Can you work these out from the model? Positions are in its coordinate system, mm. Face numbers are marked on the shaded views. A direction names the side the tool comes from. Round coordinates to 2 decimals unless told otherwise and drop trailing zeros. Loops run counter-clockwise (first coordinate to the right, second up) from the corner with the lowest first, then second, coordinate; pieces in that order, holes last. Notation, with made-up numbers: (33.25, 64) -> (53.25, 64) arc R24 cw to (53.25, 85) -> close; hole circle Ø4 at (-3.5, 52). An arc over 180 degrees is marked (long way). Answer as a JSON object with one key per item and string values.
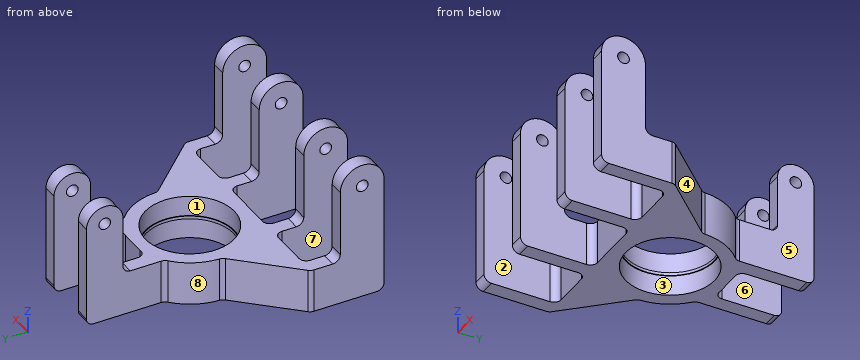
```python
from build123d import *

# Parameters (mm, degrees)
BOSS_EXTRUDE2_DEPTH     = 30
SKETCH2_R               = 4
BOSS_EXTRUDE3_DEPTH     = 10
CUT_EXTRUDE3_DEPTH      = 162
SKETCH4_R               = 4
BOSS_EXTRUDE4_DEPTH     = 10
SKETCH5_R               = 4
BOSS_EXTRUDE5_DEPTH     = 10
SKETCH6_R               = 4
BOSS_EXTRUDE6_DEPTH     = 10
SKETCH7_R               = 4
BOSS_EXTRUDE7_DEPTH     = 10
CUT_EXTRUDE4_DEPTH      = 167.226502099
CUT_EXTRUDE4_DEPTH_BACK = 57
SKETCH13_R              = 4
BOSS_EXTRUDE8_DEPTH     = 10
SKETCH14_R              = 30
CUT_EXTRUDE5_DEPTH      = 136.392946641
SKETCH15_R              = 30.5
CUT_EXTRUDE6_DEPTH      = 14
CUT_EXTRUDE7_START      = -14
SKETCH16_R              = 30.5
CUT_EXTRUDE7_DEPTH      = 14


with BuildPart() as part:
    # Sketch1 → Boss-Extrude2 (new body)
    with BuildSketch(Plane.XY):
        with BuildLine():
            Line((-15, 84.641016151), (-15, 43.789443996))
            ThreePointArc((-15, 43.789443996), (-13.139996453, 39.931036758), (-8.962922752, 38.982893886))
            Line((-8.962922752, 38.982893886), (8.962922752, 38.982893886))
            ThreePointArc((8.962922752, 38.982893886), (13.139996453, 39.931036758), (15, 43.789443996))
            Line((15, 43.789443996), (15, 84.641016151))
            Line((15, 84.641016151), (25, 84.641016151))
            Line((25, 84.641016151), (25, 33.611468644))
            ThreePointArc((25, 33.611468644), (25.447741208, 31.509528534), (26.713227694, 29.772528717))
            ThreePointArc((26.713227694, 29.772528717), (36.156075964, 17.109592948), (39.96044462, 1.778444757))
            ThreePointArc((39.96044462, 1.778444757), (40.342615834, 0.082521187), (41.289478696, -1.375443942))
            Line((41.289478696, -1.375443942), (76.166088788, -38.577161373))
            ThreePointArc((76.166088788, -38.577161373), (77.154414497, -40.136660916), (77.5, -41.950330454))
            Line((77.5, -41.950330454), (77.5, -90))
            Line((77.5, -90), (67.5, -90))
            Line((67.5, -90), (67.5, -44.931958231))
            ThreePointArc((67.5, -44.931958231), (66.055462879, -41.444537121), (62.568041769, -40))
            Line((62.568041769, -40), (37.431958231, -40))
            ThreePointArc((37.431958231, -40), (33.944537121, -41.444537121), (32.5, -44.931958231))
            Line((32.5, -44.931958231), (32.5, -90))
            Line((32.5, -90), (22.5, -90))
            Line((22.5, -90), (22.5, -44.931958231))
            ThreePointArc((22.5, -44.931958231), (21.055462879, -41.444537121), (17.568041769, -40))
            Line((17.568041769, -40), (-17.568041769, -40))
            ThreePointArc((-17.568041769, -40), (-21.055462879, -41.444537121), (-22.5, -44.931958231))
            Line((-22.5, -44.931958231), (-22.5, -90))
            Line((-22.5, -90), (-32.5, -90))
            Line((-32.5, -90), (-32.5, -44.931958231))
            ThreePointArc((-32.5, -44.931958231), (-33.944537121, -41.444537121), (-37.431958231, -40))
            Line((-37.431958231, -40), (-62.568041769, -40))
            ThreePointArc((-62.568041769, -40), (-66.055462879, -41.444537121), (-67.5, -44.931958231))
            Line((-67.5, -44.931958231), (-67.5, -90))
            Line((-67.5, -90), (-77.5, -90))
            Line((-77.5, -90), (-77.5, -41.950330454))
            ThreePointArc((-77.5, -41.950330454), (-77.154414497, -40.136660916), (-76.166088788, -38.577161373))
            Line((-76.166088788, -38.577161373), (-41.289478696, -1.375443942))
            ThreePointArc((-41.289478696, -1.375443942), (-40.342615834, 0.082521187), (-39.96044462, 1.778444757))
            ThreePointArc((-39.96044462, 1.778444757), (-36.156075964, 17.109592948), (-26.713227694, 29.772528717))
            ThreePointArc((-26.713227694, 29.772528717), (-25.447741208, 31.509528534), (-25, 33.611468644))
            Line((-25, 33.611468644), (-25, 84.641016151))
            Line((-25, 84.641016151), (-15, 84.641016151))
        make_face()
    extrude(amount=BOSS_EXTRUDE2_DEPTH)

    # Sketch2 → Boss-Extrude3 (add)
    with BuildSketch(Plane.ZY.offset(77.5)):
        with BuildLine():
            Line((30, -54.842305853), (30, -90))
            Line((30, -90), (80, -90))
            ThreePointArc((80, -90), (95, -75), (80, -60))
            Line((80, -60), (35.157694147, -60))
            ThreePointArc((35.157694147, -60), (31.51065364, -58.48934636), (30, -54.842305853))
        make_face()
        with Locations((80, -75)):
            Circle(SKETCH2_R, mode=Mode.SUBTRACT)
    extrude(amount=-BOSS_EXTRUDE3_DEPTH)

    # Sketch3 → Cut-Extrude3 (cut)
    with BuildSketch(Plane.ZY.offset(77.5)):
        with BuildLine():
            ThreePointArc((5, -90), (1.464466094, -88.535533906), (0, -85))
            Line((0, -85), (0, -90))
            Line((0, -90), (5, -90))
        make_face()
    extrude(amount=-CUT_EXTRUDE3_DEPTH, mode=Mode.SUBTRACT)

    # Sketch4 → Boss-Extrude4 (add)
    with BuildSketch(Plane.ZY.offset(32.5)):
        with BuildLine():
            Line((30, -54.842305853), (30, -90))
            Line((30, -90), (80, -90))
            ThreePointArc((80, -90), (95, -75), (80, -60))
            Line((80, -60), (35.157694147, -60))
            ThreePointArc((35.157694147, -60), (31.51065364, -58.48934636), (30, -54.842305853))
        make_face()
        with Locations((80, -75)):
            Circle(SKETCH4_R, mode=Mode.SUBTRACT)
    extrude(amount=-BOSS_EXTRUDE4_DEPTH)

    # Sketch5 → Boss-Extrude5 (add)
    with BuildSketch(Plane.ZY.offset(-22.5)):
        with BuildLine():
            Line((30, -54.842305853), (30, -90))
            Line((30, -90), (80, -90))
            ThreePointArc((80, -90), (95, -75), (80, -60))
            Line((80, -60), (35.157694147, -60))
            ThreePointArc((35.157694147, -60), (31.51065364, -58.48934636), (30, -54.842305853))
        make_face()
        with Locations((80, -75)):
            Circle(SKETCH5_R, mode=Mode.SUBTRACT)
    extrude(amount=-BOSS_EXTRUDE5_DEPTH)

    # Sketch6 → Boss-Extrude6 (add)
    with BuildSketch(Plane.ZY.offset(-67.5)):
        with BuildLine():
            Line((30, -54.842305853), (30, -90))
            Line((30, -90), (80, -90))
            ThreePointArc((80, -90), (95, -75), (80, -60))
            Line((80, -60), (35.157694147, -60))
            ThreePointArc((35.157694147, -60), (31.51065364, -58.48934636), (30, -54.842305853))
        make_face()
        with Locations((80, -75)):
            Circle(SKETCH6_R, mode=Mode.SUBTRACT)
    extrude(amount=-BOSS_EXTRUDE6_DEPTH)

    # Sketch7 → Boss-Extrude7 (add)
    with BuildSketch(Plane.ZY.offset(25)):
        with BuildLine():
            Line((70, 84.641016151), (30, 84.641016151))
            Line((30, 84.641016151), (30, 54.641016151))
            ThreePointArc((30, 54.641016151), (31.464466094, 58.176550057), (35, 59.641016151))
            Line((35, 59.641016151), (70, 59.641016151))
            ThreePointArc((70, 59.641016151), (82.5, 72.141016151), (70, 84.641016151))
        make_face()
        with Locations((70, 72.141016151)):
            Circle(SKETCH7_R, mode=Mode.SUBTRACT)
    extrude(amount=-BOSS_EXTRUDE7_DEPTH)

    # Sketch9 → Cut-Extrude4 (cut, two sides: drawn at the far end of the back side and taken through both)
    with BuildSketch(Plane.ZY.offset(25).offset(-CUT_EXTRUDE4_DEPTH_BACK)):
        with BuildLine():
            Line((0, 84.641016151), (0, 79.641016151))
            ThreePointArc((0, 79.641016151), (1.464466094, 83.176550057), (5, 84.641016151))
            Line((5, 84.641016151), (0, 84.641016151))
        make_face()
    extrude(amount=CUT_EXTRUDE4_DEPTH + CUT_EXTRUDE4_DEPTH_BACK, mode=Mode.SUBTRACT)

    # Sketch13 → Boss-Extrude8 (add)
    with BuildSketch(Plane.ZY.offset(-15)):
        with BuildLine():
            Line((70, 84.641016151), (30, 84.641016151))
            Line((30, 84.641016151), (30, 54.641016151))
            ThreePointArc((30, 54.641016151), (31.464466094, 58.176550057), (35, 59.641016151))
            Line((35, 59.641016151), (70, 59.641016151))
            ThreePointArc((70, 59.641016151), (82.5, 72.141016151), (70, 84.641016151))
        make_face()
        with Locations((70, 72.141016151)):
            Circle(SKETCH13_R, mode=Mode.SUBTRACT)
    extrude(amount=-BOSS_EXTRUDE8_DEPTH)

    # Sketch14 → Cut-Extrude5 (cut, through all)
    with BuildSketch(Plane.XY.offset(30)):
        Circle(SKETCH14_R)
    extrude(amount=-CUT_EXTRUDE5_DEPTH, mode=Mode.SUBTRACT)

    # Sketch15 → Cut-Extrude6 (cut)
    with BuildSketch(Plane.XY.offset(30)):
        Circle(SKETCH15_R)
    extrude(amount=-CUT_EXTRUDE6_DEPTH, mode=Mode.SUBTRACT)

    # Sketch16 → Cut-Extrude7 (cut)
    with BuildSketch(Plane(origin=(0, 0, 0), x_dir=(-1, 0, 0), z_dir=(0, 0, -1)).offset(CUT_EXTRUDE7_START)):
        with Locations(Location((0, 0, 0), (0, 0, 180))):
            Circle(SKETCH16_R)
    extrude(amount=CUT_EXTRUDE7_DEPTH, mode=Mode.SUBTRACT)


solid = part.part
```
Q1. I want a section at B-B, the plane x = 0. Write out the boundary of the cut face in (y, z).
Determined:
{"outline": "(-40, 0) -> (-30.5, 0) -> (-30.5, 14) -> (-30, 14) -> (-30, 16) -> (-30.5, 16) -> (-30.5, 30) -> (-40, 30) -> close; (30, 14) -> (30.5, 14) -> (30.5, 0) -> (38.98, 0) -> (38.98, 30) -> (30.5, 30) -> (30.5, 16) -> (30, 16) -> close"}
Q2. I want a section at D-D, the plane y = 27.5. Write out the boundary of the cut face in (x, z), then the cut area to 3 significant figures.
Determined:
{"outline": "(-29.05, 0) -> (-13.19, 0) -> (-13.19, 14) -> (-11.99, 14) -> (-11.99, 16) -> (-13.19, 16) -> (-13.19, 30) -> (-29.05, 30) -> close; (11.99, 14) -> (13.19, 14) -> (13.19, 0) -> (29.05, 0) -> (29.05, 30) -> (13.19, 30) -> (13.19, 16) -> (11.99, 16) -> close", "area": "956 mm²"}
Q3. On a 3-axis mill with a long thin cutter (end or side, diameter ignored), from which of +Z, -Z, +X, -X, +Y, -Y can I reach the whole of each face in a straight line? I mean the marked faces 5, 6, 7 and 8. Say none if no direction works.
Determined:
{"face 5": "+Z, -Z, +X, +Y", "face 6": "+Z, -Z, +Y", "face 7": "+Z, -Z, -Y", "face 8": "+Z, -Z, -X, +Y"}
Q4. I'm going to push flat-ended pins straight in: pin 1 (5 mm diameter, centred on x = 27, z = 54, fed in from +Y); pin 2 (12.5 mm diameter, centred on x = -49.5, z = 20.5, fed in from -Y); pin 3 (9 mm diameter, centred on y = 72.14, z = 70, fed in from -X); pin 4 (3 mm diameter, centred on x = -20.5, z = 56, fed in from -Y). Where does each tip first touch, or does it pass through?
Determined:
{"pin 1": "y = 84.64", "pin 2": "y = -40", "pin 3": "x = -25", "pin 4": "y = 59.64"}
Q5. If I drill on L1, parallel to X at y = -51, z = 17; L2, parallel to Y at x = 0, z = 10.75; L3, parallel to Y at x = 24.5, z = 51.5, over which ranges is the centre line in solid material (lowest first)? Write a range as [from, to].
Determined:
{"L1": "[-77.5, -67.5], [-32.5, -22.5], [22.5, 32.5], [67.5, 77.5]", "L2": "[-40, -30.5], [30.5, 38.98]", "L3": "[-90, -60], [59.64, 84.64]"}
Q6. I want a section at A-A, the plane y = 46. Write out the boundary of the cut face in (x, z).
Determined:
{"outline": "(-25, 0) -> (-15, 0) -> (-15, 30) -> (-25, 30) -> close; (15, 0) -> (25, 0) -> (25, 30) -> (15, 30) -> close"}
Q7. We'd pull the mould along Y, two halves only. Please class the marked faces 1, 2, 3 and 4: pulls with the +Y half, pulls with the -Y half, needs draft (parallel to the pull), parting line crosses it, or undercut.
Determined:
{"face 1": "undercut", "face 2": "needs draft", "face 3": "undercut", "face 4": "pulls with the +Y half"}
Q8. I want a section at C-C, the plane y = -75. Give the number of separate pieces and of enclosed holes in the cut face, then the cut area to 3 significant figures.
Determined:
{"separate pieces": "8", "enclosed holes": "0", "area": "3,480 mm²"}
